Here's how the part is built. I have some questions about the finished solid (model axes, mm). Face numbers are marked on the shaded views. A direction names the side the tool comes from. Coordinates: 2 decimals unless noted, no trailing zeros. Write each loop counter-clockwise with the first axis right and the second up, starting at its lowest first coordinate (ties: lowest second). Pieces come first, ordered by that corner, then holes.
(1) Please list where these lines run through material, in increasing order: probe 1 along Z at (x, y) = (164, 20.45); probe 2 along X at (y, z) = (19.95, 172); probe 3 along X at (y, z) = (3.5, 143.5).
(2) For pin 1 Ø3 at (y, z) = (17.5, 112.5) entering from -X; pin 2 Ø3 at (x, z) = (65, 172.5) entering from +Y, each with a flat end and sliding along its axis, tell me the tip position at first contact or that it passes through.
(3) Imagine slicing it at B-B, the plane z = 131.5. List the corners of the cut face in (x, y) for me.
(4) Imagine slicing it at A-A, the plane x = 136. List the corners of the cut face in (y, z) for me.
(5) Which directions (+Z, -Z, +X, -X, +Y, -Y) give clear straight access to the entire face, cutting with the end or side of a thin tool? Please do the marked faces 1 and 2.
(6) Imagine slicing it at C-C, the plane y = 12.75. List the corners of the cut face in (x, z) for me, plus the area to 3 significant figures.
(7) Thinking about a two-plate mould opening in Z: for the marked faces 3, 4 and 5, which applies, released by +Z, released by -Z, zero draft, split by the parting line, or undercut?
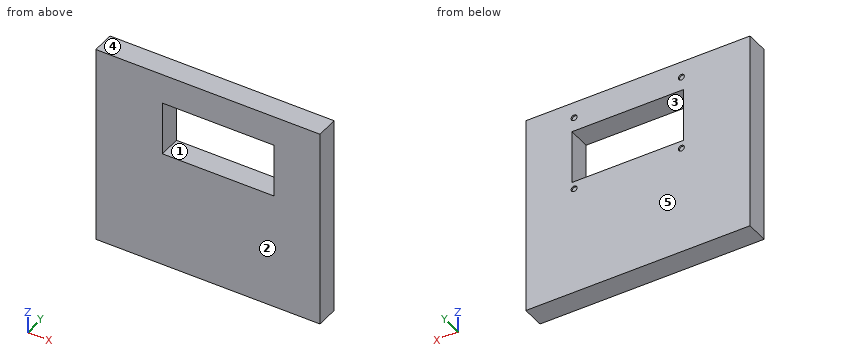
Autodesk Fusion 360 part; units mm, degrees
sketch "Smartie Feed Support" plane through (0, 0, 0) normal (0, 0, 1) x (1, 0, 0)
  line L0 (0, 0) -> (209, 0)
  line L1 (209, 0) -> (209, 21)
  line L2 (209, 21) -> (0, 21)
  line L3 (0, 21) -> (0, 0)
  dimension "d1" = 209
  dimension "d2" = 21
extrude "Extrude1" add sketch "Smartie Feed Support" along normal blind 187
sketch "Outlet" plane through (0, 0, 0) normal (0, -1, 0) x (1, 0, 0)
  line L0 (0, 0) -> (209, 0)
  line L1 (209, 0) -> (209, 187)
  line L2 (209, 187) -> (0, 187)
  line L3 (0, 187) -> (0, 0)
  line L4 (69, 146) -> (159, 146)
  line L5 (159, 146) -> (159, 116)
  line L6 (159, 116) -> (69, 116)
  line L7 (69, 116) -> (69, 146)
  dimension "d31" = 30
  dimension "d32" = 90
  dimension "d33" = 69
  dimension "d34" = 50
  dimension "d35" = 41
sketch "Inlet" plane through (0, 21, 0) normal (0, 1, 0) x (-1, 0, 0)
  line L0 (-209, 0) -> (0, 0)
  line L1 (0, 0) -> (0, 187)
  line L2 (0, 187) -> (-209, 187)
  line L3 (-209, 187) -> (-209, 0)
  line L4 (-69, 152) -> (-159, 152)
  line L5 (-159, 152) -> (-159, 122)
  line L6 (-159, 122) -> (-69, 122)
  line L7 (-69, 122) -> (-69, 152)
  dimension "d36" = 90
  dimension "d37" = 69
  dimension "d38" = 30
  dimension "d39" = 35
  dimension "d40" = 50
loft "Loft9" cut profiles "Inlet", "Outlet" section 1 contours L4 L5 L6 L7 section 2 contours L4 L5 L6 L7
sketch "Magnet Holes" plane through (0, 21, 0) normal (0, 1, 0) x (-1, 0, 0)
  line L0 (-69, 152) -> (-69, 122)
  line L1 (-69, 122) -> (-159, 122)
  line L2 (-159, 122) -> (-159, 152)
  line L3 (-159, 152) -> (-69, 152)
  line L4 (-209, 0) -> (0, 0)
  line L5 (0, 0) -> (0, 187)
  line L6 (0, 187) -> (-209, 187)
  line L7 (-209, 187) -> (-209, 0)
  circle A0 centre (-164, 172) radius 2.75
  circle A1 centre (-64, 172) radius 2.75
  circle A2 centre (-164, 102) radius 2.75
  circle A3 centre (-64, 102) radius 2.75
  dimension "d43" = 5.5
  dimension "d44" = 5.5
  dimension "d45" = 5.5
  dimension "d46" = 5.5
  dimension "d49" = 64
  dimension "d50" = 64
  dimension "d51" = 164
  dimension "d52" = 164
  dimension "d53" = 20
  dimension "d54" = 20
  dimension "d55" = 20
  dimension "d56" = 20
extrude "Extrude2" cut sketch "Magnet Holes" against normal blind 1.5 contours A0 | A1 | A2 | A3
sketch "Separator" plane through (0, 21, 0) normal (0, 1, 0) x (-1, 0, 0)
  circle A0 centre (-164, 102) radius 2.75
  circle A1 centre (-64, 172) radius 2.75
  circle A2 centre (-164, 172) radius 2.75
  circle A3 centre (-64, 102) radius 2.75
  line L0 (-69, 152) -> (-69, 122)
  line L1 (-69, 122) -> (-159, 122)
  line L2 (-159, 122) -> (-159, 152)
  line L3 (-159, 152) -> (-69, 152)
  line L4 (-209, 0) -> (0, 0)
  line L5 (0, 0) -> (0, 187)
  line L6 (0, 187) -> (-209, 187)
  line L7 (-209, 187) -> (-209, 0)
  line L8 (-159, 152) -> (-69, 152)
  line L9 (-69, 152) -> (-69, 122)
  line L10 (-159, 122) -> (-159, 152)
  line L11 (-159, 116) -> (-69, 116)
  line L12 (-159, 146) -> (-159, 116)
  line L13 (-69, 116) -> (-69, 146)
  line L14 (-69, 146) -> (-159, 146)
  line L15 (-69, 122) -> (-159, 122)
  line L16 (-166, 159) -> (-62, 159)
  line L17 (-62, 159) -> (-62, 109)
  line L18 (-62, 109) -> (-166, 109)
  line L19 (-166, 109) -> (-166, 159)
  dimension "d57" = 7
  dimension "d58" = 7
  dimension "d59" = 7
  dimension "d60" = 7
extrude "Extrude3" cut sketch "Separator" against normal blind 21 contours L0 L2 L3 L8 L9 L10 L14 | L0 L1 L2 L9 L10 L12 L13 L14 L15 | L1 L11 L12 L13 L15 | L16 L17 L18 L19
equation "d1 = 219 mm - 10 mm"
equation "d3 = 166 mm + 21 mm"
equation "outletHeight = 15 mm"
equation "outletWidth = 20 mm"
equation "sortedContainersMidpointWidth = sortedContainersWidth + polycarbonateThickness"
equation "sortedContainersWidth = 60 mm"
equation "sortedContainersHeight = 113 mm"
equation "polycarbonateThickness = 6 mm"
equation "sortedContainersMidpointHeight = sortedContainersHeight + polycarbonateThickness"
equation "d33 = 90 mm - 21 mm"
equation "d35 = 30 mm - 21 mm + 5 mm + 6 mm + 21 mm"
equation "d37 = 90 mm - 21 mm"
equation "d39 = 30 mm - 21 mm + 5 mm + 21 mm"
equation "magnetDiameter = 5 mm"
equation "magnetHeight = 1.5 mm"
equation "d43 = magnetDiameter + 0.5 mm"
equation "d44 = magnetDiameter + 0.5 mm"
equation "d45 = magnetDiameter + 0.5 mm"
equation "d46 = magnetDiameter + 0.5 mm"
equation "d49 = 75 mm - 21 mm + 10 mm"
equation "d50 = 75 mm - 21 mm + 10 mm"
equation "d51 = 195 mm - 10 mm - 21 mm"
equation "d52 = 195 mm - 10 mm - 21 mm"
Recorded:
1. probe 1: z = 0 to 99.25, 104.75 to 109, 159 to 169.25, 174.75 to 187
1. probe 2: x = 0 to 61.25, 66.75 to 161.25, 166.75 to 209
1. probe 3: x = 0 to 62, 166 to 209
2. pin 1: stops at x = 0
2. pin 2: stops at y = 19.5
3. outline: (0, 0) - (62, 0) - (62, 21) - (0, 21) - close; (166, 0) - (209, 0) - (209, 21) - (166, 21) - close
4. outline: (0, 0) - (21, 0) - (21, 109) - (0, 109) - close; (0, 159) - (21, 159) - (21, 187) - (0, 187) - close
5. face 1: +Y, -Y
5. face 2: +Z, -Z, +X, -X, -Y
6. outline: (0, 0) - (209, 0) - (209, 187) - (0, 187) - close; hole (62, 109) - (166, 109) - (166, 159) - (62, 159) - close
6. area: 33,900 mm2
7. face 3: undercut
7. face 4: released by +Z
7. face 5: zero draft
